from build123d import *

# Parameters (mm, degrees)
SKETCH_1_W            = 103.2
SKETCH_1_H            = 20
EXTRUDE_1_DEPTH       = 39.7
SKETCH_2_W            = 88.2
SKETCH_2_H            = 33.7
CUT_EXTRUDE_1_DEPTH   = 17
EXTRUDE_START         = -3
SKETCH_3_W            = 30
SKETCH_3_H            = 50
EXTRUDE_2_DEPTH       = 29
SKETCH_21_W           = 20.2
SKETCH_21_H           = 20.2
CUT_EXTRUDE_11_DEPTH  = 30.15
SKETCH_22_W           = 20.2
SKETCH_22_H           = 50
CUT_EXTRUDE_12_DEPTH  = 3.65
CUT_EXTRUDE_14_DEPTH  = 88.244254825
EXTRUDE_4_DEPTH       = 3
F_2_5MM_2_D           = 2.5
F_2_5MM_2_CSINK_D     = 2.55
F_2_5MM_2_CSINK_ANGLE = 90
F_5_0MM_3_D           = 5
F_5_0MM_3_DEPTH       = 3
F_5_0MM_3_CSINK_D     = 5.05
F_5_0MM_3_CSINK_ANGLE = 90
SKETCH_30_W           = 52.520858891
SKETCH_30_H           = 19.35
CUT_EXTRUDE_15_DEPTH  = 1.9
CUT_EXTRUDE_16_DEPTH  = 1.9
F_5_0MM_4_D           = 5
F_5_0MM_4_CSINK_D     = 5.05
F_5_0MM_4_CSINK_ANGLE = 90
CUT_EXTRUDE_19_DEPTH  = 118.585033061
F_2_5MM_1_D           = 2.5
F_2_5MM_1_CSINK_D     = 2.55
F_2_5MM_1_CSINK_ANGLE = 90


with BuildPart() as part:
    # 草图1 → 凸台-拉伸1 (new body)
    with BuildSketch(Plane.XY):
        with Locations((-51.6, 10)):
            Rectangle(SKETCH_1_W, SKETCH_1_H)
    extrude(amount=EXTRUDE_1_DEPTH)

    # 草图2 → 切除-拉伸1 (cut)
    with BuildSketch(Plane(origin=(0, 20, 0), x_dir=(1, 0, 0), z_dir=(0, 1, 0))):
        with Locations((-51.6, -19.85)):
            Rectangle(SKETCH_2_W, SKETCH_2_H)
    extrude(amount=-CUT_EXTRUDE_1_DEPTH, mode=Mode.SUBTRACT)

    # 草图3 → 凸台-拉伸2 (add)
    with BuildSketch(Plane.XZ.offset(EXTRUDE_START)):
        with Locations((-51.6, 25)):
            Rectangle(SKETCH_3_W, SKETCH_3_H)
    extrude(amount=EXTRUDE_2_DEPTH)

    # 草图21 → 切除-拉伸11 (cut)
    with BuildSketch(Plane.XY.offset(50)):
        with Locations((-51.6, -9.25)):
            Rectangle(SKETCH_21_W, SKETCH_21_H)
    extrude(amount=-CUT_EXTRUDE_11_DEPTH, mode=Mode.SUBTRACT)

    # 草图22 → 切除-拉伸12 (cut)
    with BuildSketch(Plane.XZ.offset(26)):
        with Locations((-51.6, 25)):
            Rectangle(SKETCH_22_W, SKETCH_22_H)
    extrude(amount=-CUT_EXTRUDE_12_DEPTH, mode=Mode.SUBTRACT)

    # 草图24 → 切除-拉伸14 (cut, through all)
    with BuildSketch(Plane(origin=(-36.6, 0, 0), x_dir=(0, 0, -1), z_dir=(1, 0, 0))):
        Polygon((0, 0), (0, -26), (-19.85, -26), align=None)
    extrude(amount=-CUT_EXTRUDE_14_DEPTH, mode=Mode.SUBTRACT)

    # 草图25 → 凸台-拉伸4 (add)
    with BuildSketch(Plane.XZ):
        Polygon((-36.6, 39.7), (-36.6, 50), (0, 39.7), align=None)
        Polygon((-66.6, 39.7), (-103.2, 39.7), (-66.6, 50), align=None)
    extrude(amount=-EXTRUDE_4_DEPTH)

    # Ø2.5mm 暗销孔2 (through all)
    with Locations(Plane(origin=(0, 0, 0), x_dir=(-1, 0, 0), z_dir=(0, 0, -1))):
        with Locations((81.6, 9.75), (37.6, 9.75), (21.6, 9.75), (65.6, 9.75)):
            CounterSinkHole(F_2_5MM_2_D / 2, F_2_5MM_2_CSINK_D / 2, counter_sink_angle=F_2_5MM_2_CSINK_ANGLE)

    # Ø5.0mm 暗销孔3
    with Locations(Plane(origin=(0, -22.35, 0), x_dir=(-1, 0, 0), z_dir=(0, -1, 0))):
        with Locations((51.6, -40.85), (51.6, -25.85)):
            CounterSinkHole(F_5_0MM_3_D / 2, F_5_0MM_3_CSINK_D / 2, depth=F_5_0MM_3_DEPTH, counter_sink_angle=F_5_0MM_3_CSINK_ANGLE)

    # 草图30 → 切除-拉伸15 (cut)
    with BuildSketch(Plane(origin=(-36.6, 0, 0), x_dir=(0, 0, -1), z_dir=(1, 0, 0))):
        with Locations((-23.739570554, -9.675)):
            Rectangle(SKETCH_30_W, SKETCH_30_H)
    extrude(amount=-CUT_EXTRUDE_15_DEPTH, mode=Mode.SUBTRACT)

    # 草图31 → 切除-拉伸16 (cut)
    with BuildSketch(Plane.ZY.offset(66.6)):
        Polygon((0, 0), (14.772980769, -19.35), (50, -19.35), (50, 0), align=None)
    extrude(amount=-CUT_EXTRUDE_16_DEPTH, mode=Mode.SUBTRACT)

    # Ø5.0mm 暗销孔4 (through all)
    with Locations(Plane(origin=(-38.5, 0, 0), x_dir=(0, 0, -1), z_dir=(1, 0, 0))):
        with Locations((-25.85, -9.25)):
            CounterSinkHole(F_5_0MM_4_D / 2, F_5_0MM_4_CSINK_D / 2, counter_sink_angle=F_5_0MM_4_CSINK_ANGLE)

    # 草图35 → 切除-拉伸19 (cut, through all)
    with BuildSketch(Plane(origin=(0, 0, 0), x_dir=(-1, 0, 0), z_dir=(0, 0, -1))):
        Polygon((103.2, 20), (81.6, 20), (103.2, 9.75), align=None)
        Polygon((0, 20), (0, 9.75), (21.6, 20), align=None)
        Polygon((65.6, 20), (51.6, 15), (37.6, 20), align=None)
    extrude(amount=-CUT_EXTRUDE_19_DEPTH, mode=Mode.SUBTRACT)

    # Ø2.5mm 暗销孔1 (through all)
    with Locations(Plane(origin=(0, 0, 0), x_dir=(-1, 0, 0), z_dir=(0, 0, -1))):
        with Locations((81.6, 9.75), (37.6, 9.75), (21.6, 9.75), (65.6, 9.75)):
            CounterSinkHole(F_2_5MM_1_D / 2, F_2_5MM_1_CSINK_D / 2, counter_sink_angle=F_2_5MM_1_CSINK_ANGLE)


solid = part.part
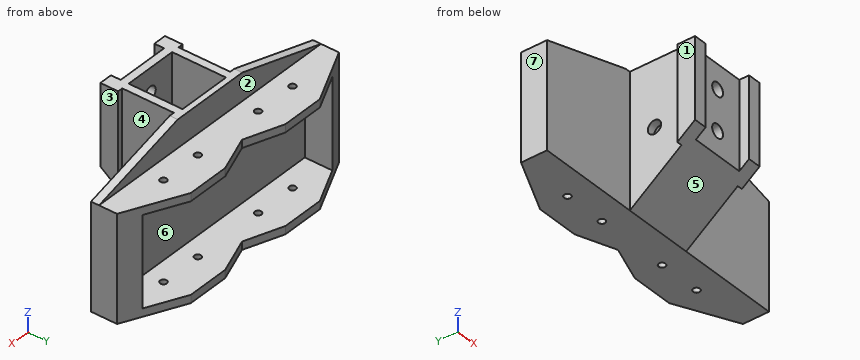
Could you check a few things on this model? Use its own coordinates, in mm. Face numbers are marked on the shaded views. A direction names the side the tool comes from. Round coordinates to 2 decimals unless told otherwise and drop trailing zeros. Order: outer loops, then holes, each group sorted by start corner. A loop starts at its lowest first (then second) coordinate and runs counter-clockwise, first axis right, second up.
Q1. I'm going to push flat-ended pins straight in: P1, Ø5, axis at x = -48, y = -13, coming from the -Z side; P2, Ø13.5, axis at x = -39.5, y = 13, coming from the +Z side; P3, Ø1.5, axis at x = -54, z = 37, coming from the +Y side (3 decimals); P4, Ø21.5, axis at y = -10, z = 22.5, coming from the +X side. Where does each tip first touch, or does it pass through?
Geometry says:
P1: stops at z = 8.02
P2: stops at z = 39.7
P3: stops at y = 16.125
P4: stops at x = 0
Q2. Imagine slicing it at D-D, the plane z = 40.85. List the corners of the cut face in (x, y) for me (3 decimals), then the cut area to 3 significant figures.
Geometry says:
outline: (-99.114, 0) - (-64.7, 0) - (-64.7, -19.35) - (-66.6, -19.35) - (-66.6, -26) - (-61.7, -26) - (-61.7, -22.35) - (-54.125, -22.35) - (-54.1, -22.325) - (-54.1, -19.35) - (-61.7, -19.35) - (-61.7, 0.85) - (-41.5, 0.85) - (-41.5, -19.35) - (-49.1, -19.35) - (-49.1, -22.325) - (-49.075, -22.35) - (-41.5, -22.35) - (-41.5, -26) - (-36.6, -26) - (-36.6, -19.35) - (-38.5, -19.35) - (-38.5, 0) - (-4.086, 0) - (-4.086, 3) - (-99.114, 3) - close
area: 495 mm2
Q3. Imagine slicing it at A-A, the plane z = 35. List the corners of the cut face in (x, y) for me.
Geometry says:
outline: (-103.2, 0) - (-64.7, 0) - (-64.7, -19.35) - (-66.6, -19.35) - (-66.6, -26) - (-61.7, -26) - (-61.7, -22.35) - (-41.5, -22.35) - (-41.5, -26) - (-36.6, -26) - (-36.6, -19.35) - (-38.5, -19.35) - (-38.5, 0) - (0, 0) - (0, 9.75) - (-7.5, 13.31) - (-7.5, 3) - (-95.7, 3) - (-95.7, 13.31) - (-103.2, 9.75) - close; hole (-61.7, -19.35) - (-41.5, -19.35) - (-41.5, 0.85) - (-61.7, 0.85) - close
Q4. Which directions (+Z, -Z, +X, -X, +Y, -Y) give clear straight access to the entire face, cutting with the end or side of a thin tool? Please do the marked faces 1, 2, 3 and 4.
Geometry says:
face 1: +Z, -Z, -X, -Y
face 2: +Z, +X, -X, +Y
face 3: +Z, -Z, +X, -Y
face 4: +Z, -Z, +X
Q5. Thinking about a two-plate mould opening in Z: for the marked faces 5, 6 and 7, which applies, released by +Z, released by -Z, zero draft, split by the parting line, or undercut?
Geometry says:
face 5: released by -Z
face 6: undercut
face 7: zero draft
Q6. Imagine slicing it at B-B, the plane y = -9.25. List the corners of the cut face in (x, z) for me (3 decimals).
Geometry says:
outline: (-64.7, 7.062) - (-38.5, 7.062) - (-38.5, 23.325) - (-38.525, 23.35) - (-41.5, 23.35) - (-41.5, 19.85) - (-61.7, 19.85) - (-61.7, 23.35) - (-64.7, 23.35) - close; (-64.7, 28.35) - (-61.7, 28.35) - (-61.7, 50) - (-64.7, 50) - close; (-41.5, 28.35) - (-38.525, 28.35) - (-38.5, 28.375) - (-38.5, 50) - (-41.5, 50) - close
Q7. Imagine slicing it at C-C, the plane x = -29.5. List the corners of the cut face in (y, z) for me.
Geometry says:
outline: (0, 0) - (20, 0) - (20, 3) - (3, 3) - (3, 36.7) - (20, 36.7) - (20, 39.7) - (3, 39.7) - (3, 48) - (0, 48) - close
Q8. Please list where these lines run through material, in increasing order: probe 1 along X at (y, z) = (9.75, 1.65); probe 2 along X at (y, z) = (-18.5, 47.5); probe 3 along Z at (x, y) = (-88, 4.5).
Geometry says:
probe 1: x = -103.2 to -82.85, -80.35 to -66.85, -64.35 to -38.85, -36.35 to -22.85, -20.35 to 0
probe 2: x = -64.7 to -61.7, -41.5 to -38.5
probe 3: z = 0 to 3, 36.7 to 39.7
